Can you work these out from the drawing? Everything is in mm from the part's minimum corner. Coordinates: 2 decimals unless noted, no trailing zeros. Loops run counter-clockwise (first coordinate to the right, second up) from the corner with the lowest first, then second, coordinate; pieces in that order, holes last. Notation, with made-up numbers: M 69,31 L 90,31 A18 ccw 90,64 Z; hole C 30,74 d3. An arc over 180 degrees is marked long. Use CSV: the item, a comma, the result in double quotes. Start each with the question number.
Q1. If we section it at D-D (x = 25.4): Please give me the cut outline in (y, z).
Q2. If we section it at A-A (x = 88.9): Please give me the cut outline in (y, z).
Q3. If we section it at C-C (y = 9.5): Please give me the cut outline in (x, z), and give its area (3 significant figures).
Q4. If we section it at B-B (x = 6.35): Please give me the cut outline in (y, z), and give its area (3 significant figures).
Q5. Please list where these lines run through material, in increasing order: probe 1 along Y at (x, z) = (6.35, 8.25); probe 2 along X at (y, z) = (49, 9) (1 decimal); probe 3 along Y at (x, z) = (25.4, 9.25). Write a range as [from, to].
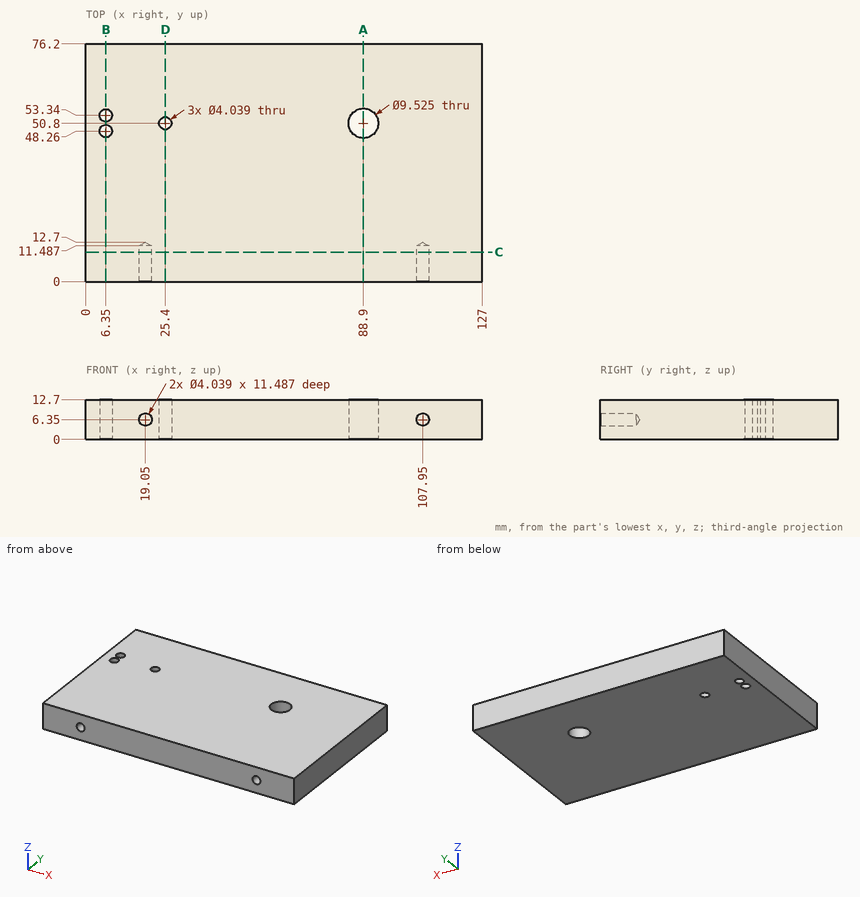
Results below:
1,outline,"M 0,0 L 48.78,0 L 48.78,12.7 L 0,12.7 Z; M 52.82,0 L 76.2,0 L 76.2,12.7 L 52.82,12.7 Z"
2,outline,"M 0,0 L 46.04,0 L 46.04,12.7 L 0,12.7 Z; M 55.56,0 L 76.2,0 L 76.2,12.7 L 55.56,12.7 Z"
3,outline,"M 0,0 L 127,0 L 127,12.7 L 0,12.7 Z; hole C 19.05,6.35 d4.04; hole C 107.95,6.35 d4.04"
3,area,"1,590 mm^2"
4,outline,"M 0,0 L 46.24,0 L 46.24,12.7 L 0,12.7 Z; M 50.28,0 L 51.32,0 L 51.32,12.7 L 50.28,12.7 Z; M 55.36,0 L 76.2,0 L 76.2,12.7 L 55.36,12.7 Z"
4,area,"865 mm^2"
5,probe 1,"[0, 46.24], [50.28, 51.32], [55.36, 76.2]"
5,probe 2,"[0, 4.5], [8.2, 24.5], [26.3, 84.5], [93.3, 127]"
5,probe 3,"[0, 48.78], [52.82, 76.2]"
